Study the drawing (mm; zero at the part's minimum x, y, z) and answer. Coordinates: 2 decimals unless noted, no trailing zeros. Order: outer loops, then holes, each group sorted by start corner. A loop starts at its lowest first (then second) coordinate and runs counter-clockwise, first axis right, second up. Notation, with made-up numbers: (28.5, 23) -> (49.5, 23) arc R20 cw to (49.5, 61) -> close; hole circle Ø8 at (-38, 86.5). An arc over 180 degrees is marked (long way). Write each question's results on one line, items separated by ' | '. Start each with the question number.
(1) The part is cut by section C-C, the plane z = 102. Give the vertices of the cut face in (x, y).
(2) Given pin 1 (12.5 mm diameter, centred on x = 140, z = 140, fed in from +Y), flat-ended and moving along its own axis, determine where the tip first touches the part or whether it passes through.
(3) The part is cut by section A-A, the plane z = 13. Count the separate pieces of the cut face and the enclosed holes in it, then the cut area to 3 significant figures.
(4) Straight lines are drawn through the part: L1, parallel to X at y = 2.75, z = 140; L2, parallel to X at y = 2.75, z = 117.6; L3, parallel to Z at x = 105, y = 3.5 (1 decimal). For each, find the intervals that lie inside material, in ascending order.
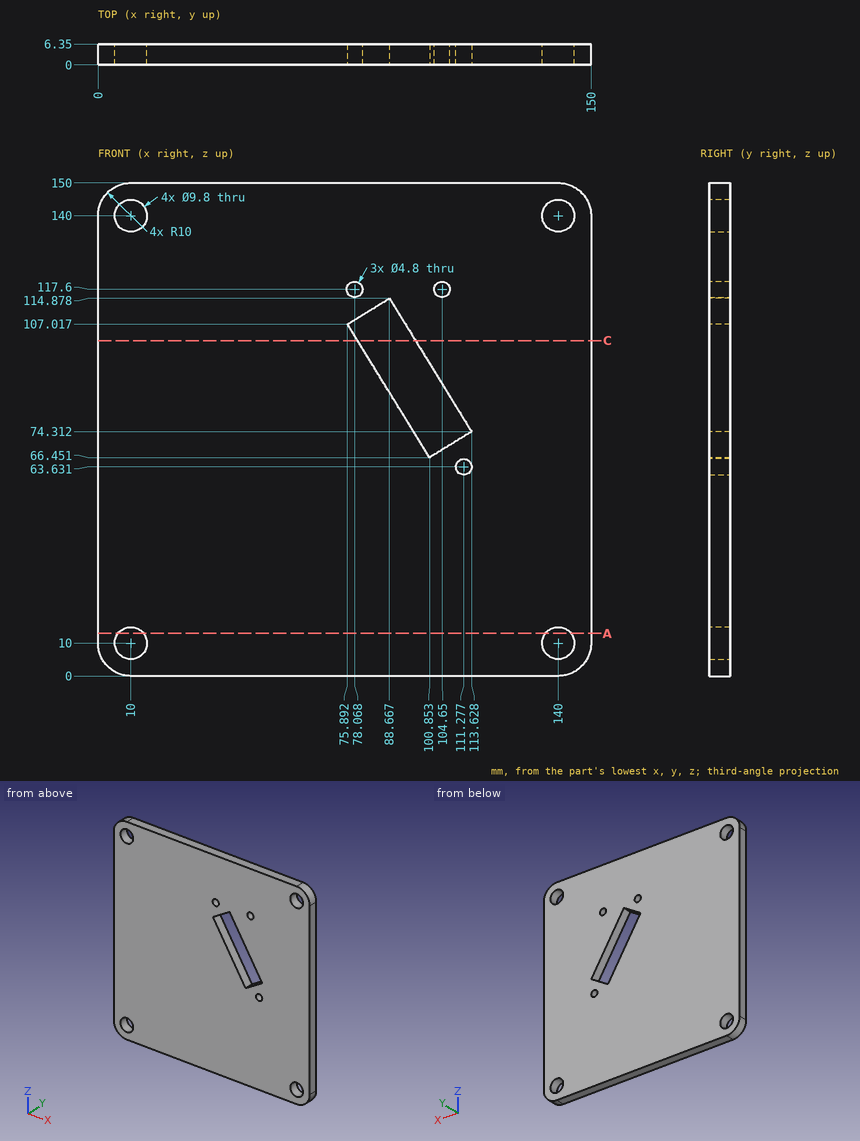
Established:
1) outline: (0, 0) -> (78.98, 0) -> (78.98, 6.35) -> (0, 6.35) -> close; (96.59, 0) -> (150, 0) -> (150, 6.35) -> (96.59, 6.35) -> close
2) pin 1: stops at y = 6.35
3) separate pieces: 3 | enclosed holes: 0 | area: 854 mm^2
4) L1: x = 0 to 5.1, 14.9 to 135.1, 144.9 to 150 | L2: x = 0 to 75.67, 80.47 to 102.25, 107.05 to 150 | L3: z = 0 to 69, 88.3 to 115.2, 120 to 150
